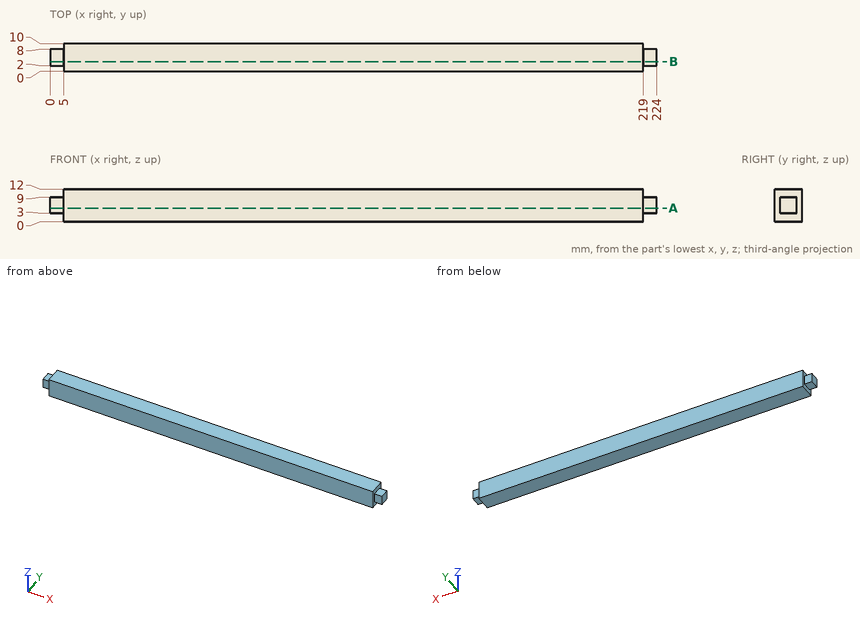
The drawing under review shows one solid part. Ordinate dimensions are in mm from its lowest x, y, z. Round coordinates to 2 decimals unless told otherwise and drop trailing zeros. Write each loop counter-clockwise with the first axis right and the second up, starting at its lowest first coordinate (ties: lowest second). Pieces come first, ordered by that corner, then holes. Notation, with made-up numbers: M 43.25,11 L 88.25,11 A32 ccw 88.25,45 Z; hole C 17.25,-15 d4. An arc over 180 degrees is marked long. One line per item, written item: value. Start each with the question number.
(1) We need section A-A (z = 5). Give the boundary of the cut face in (x, y), and give its area (3 significant figures).
(2) Insertion check: pin 1 (1.5 mm diameter, centred on x = 222.5, y = 4, fed in from +Z); pin 2 (2.5 mm diameter, centred on x = 221.5, y = 4, fed in from -Z); pin 3 (2 mm diameter, centred on y = 4, z = 11, fed in from +X). Each pin has a flat end and moves straight along its axis. Give the tip position at first contact, or say it passes through.
(3) Wall thickness on line 1 (X direction, y = 6, z = 2): over which ranges is the line inside the solid? List them lowest first.
(4) We need section B-B (y = 3.5). Give the boundary of the cut face in (x, z), and give its area (3 significant figures).
Result:
1. outline: M 0,2 L 5,2 L 5,0 L 219,0 L 219,2 L 224,2 L 224,8 L 219,8 L 219,10 L 5,10 L 5,8 L 0,8 Z
1. area: 2,200 mm²
2. pin 1: z = 9
2. pin 2: z = 3
2. pin 3: x = 219
3. line 1: 5 to 219
4. outline: M 0,3 L 5,3 L 5,0 L 219,0 L 219,3 L 224,3 L 224,9 L 219,9 L 219,12 L 5,12 L 5,9 L 0,9 Z
4. area: 2,630 mm²
